Build history of the part. All positions in model axes, mm. Round coordinates to 2 decimals unless told otherwise and drop trailing zeros. Write each loop counter-clockwise with the first axis right and the second up, starting at its lowest first coordinate (ties: lowest second). Pieces come first, ordered by that corner, then holes.
Item 1: Drop flat-ended pins along their axis: pin 1 Ø6 at (x, z) = (-22.5, 6.5) entering from +Y; pin 2 Ø6 at (y, z) = (399.5, 8.5) entering from +X; pin 3 Ø3 at (x, z) = (-120, 3) entering from +Y. Give the stop position or say it passes through.
Item 2: Band-saw the part on B-B, the plane y = 146.5. Count the separate pieces of the cut face and the enclosed holes in it, then the cut area to 3 significant figures.
Item 3: Wall check: probe 1 along X at (y, z) = (111, 5.5); probe 2 along Z at (x, y) = (-216.5, 96.5); probe 3 along X at (y, z) = (102, -3.25). Give the ranges that are in metal, low to high.
Item 4: Band-saw the part on A-A, the plane z = 2.75. Write the cut outline in (x, y), then the cut area to 3 significant figures.
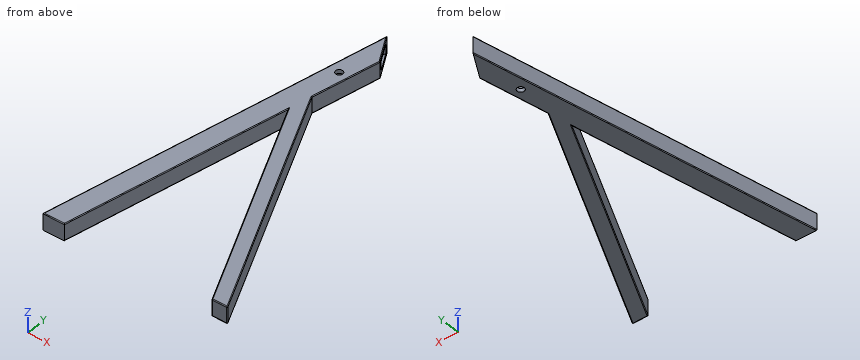
```python
from build123d import *

# Parameters (mm, degrees)
BOSS_EXTRUDE2_DEPTH = 11.75
CUT_EXTRUDE1_DEPTH  = 6.5
SKETCH3_R           = 5
CUT_EXTRUDE2_DEPTH  = 540.96055804
FILLET2_R           = 1


with BuildPart() as part:
    # Sketch1 → Boss-Extrude2 (new, symmetric)
    with BuildSketch(Plane.XY):
        Polygon((-154.033564487, 314.282772375), (-148.14056714, 347.703621092), (22.272935761, 0), (0, 0), align=None)
        Polygon((-154.718136007, 483.163488855), (-239.912895185, 0), (-209.450096828, 0), (-131.308416878, 443.163488855), align=None)
    extrude(amount=BOSS_EXTRUDE2_DEPTH, both=True)

    # Sketch2 → Cut-Extrude1 (cut, symmetric)
    with BuildSketch(Plane.XY):
        Polygon((-234.483108164, 2), (-214.174575926, 2), (-126.011085572, 502), (-139.266538582, 542), align=None)
    extrude(amount=CUT_EXTRUDE1_DEPTH, both=True, mode=Mode.SUBTRACT)

    # Sketch3 → Cut-Extrude2 (cut, through all)
    with BuildSketch(Plane.XY.offset(11.75)):
        with Locations((-153.135277111, 400)):
            Circle(SKETCH3_R)
    extrude(amount=-CUT_EXTRUDE2_DEPTH, mode=Mode.SUBTRACT)

    # Fillet2
    fillet2_edges = [part.edges().sort_by_distance(p)[0] for p in [
        (-62.933815689, 173.851810546, -11.75),
        (11.136467881, 0, 11.75),
        (-77.016782243, 157.141386187, 11.75),
        (-181.741830658, 157.141386187, 11.75),
        (-224.681496007, 0, 11.75),
        (-197.315515596, 241.581744428, 11.75),
        (-143.013276442, 463.163488855, 11.75),
        (-139.724492009, 395.433554974, 11.75),
        (-62.933815689, 173.851810546, 11.75),
        (11.136467881, 0, -11.75),
        (-77.016782243, 157.141386187, -11.75),
        (0, 0, 0),
        (22.272935761, 0, 0),
        (-148.14056714, 347.703621092, 0),
        (-181.741830658, 157.141386187, -11.75),
        (-197.315515596, 241.581744428, -11.75),
        (-139.724492009, 395.433554974, -11.75),
    ]]
    fillet(fillet2_edges, radius=FILLET2_R)


solid = part.part
```
Results:
1. pin 1: stops at y = 97.47
1. pin 2: stops at x = -138.48
1. pin 3: stops at y = 293.35
2. separate pieces: 2
2. enclosed holes: 1
2. area: 973 mm2
3. probe 1: x = -220.34 to -215.26, -194.95 to -189.88, -54.4 to -32.13
3. probe 2: z = -11.75 to -6.5, 6.5 to 11.75
3. probe 3: x = -221.93 to -216.85, -196.54 to -191.46, -49.99 to -27.72
4. outline: (-239.91, 0) - (-209.45, 0) - (-154.03, 314.28) - (-0.27, 0.56) arc R1 ccw to (0.62, 0) - (20.67, 0) arc R1 ccw to (21.57, 1.44) - (-148, 347.41) arc R1 cw to (-148.08, 348.02) - (-131.31, 443.16) - (-135.21, 449.83) - (-214.17, 2) - (-234.48, 2) - (-150.82, 476.5) - (-154.72, 483.16) - close
4. area: 12,100 mm2
